Check sheet for the modelled part. Datum: model origin and axes. Units: mm. Round coordinates to 2 decimals unless told otherwise and drop trailing zeros. Write each loop counter-clockwise with the first axis right and the second up, starting at its lowest first coordinate (ties: lowest second). Pieces come first, ordered by that corner, then holes. Notation, with made-up numbers: (17.5, -14.5) -> (24.5, -14.5) arc R8 ccw to (24.5, -4.5) -> close; hole circle Ø2 at (44, 6.5). An arc over 180 degrees is marked (long way). One line per item, written item: value.
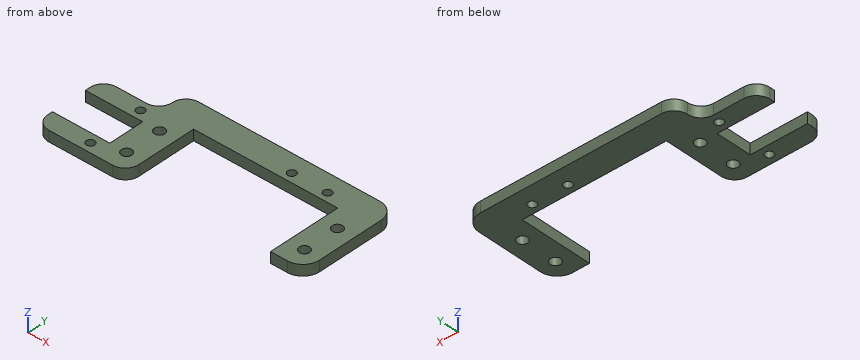
from build123d import *

# Parameters (mm, degrees)
BOSS_EXTRUDE7_DEPTH = 3
SKETCH12_R          = 1.15
CUT_EXTRUDE3_DEPTH  = 70.389048127
SKETCH11_R          = 1.45
CUT_EXTRUDE4_DEPTH  = 70.389048127
SKETCH13_R          = 1.15
CUT_EXTRUDE5_DEPTH  = 70.389048127
FILLET1_R           = 4.7
FILLET2_R           = 3.8


with BuildPart() as part:
    # Sketch10 → Boss-Extrude7 (new body)
    with BuildSketch(Plane.XY):
        Polygon((17.4, 10.2), (57.6, 10.2), (57.6, -10.2), (67, -10.2), (67, 17.8), (8, 17.8), (8, 10.2), (-8, 10.2), (-8, 5), (8, 5), (8, -5), (-8, -5), (-8, -10.2), (17.4, -10.2), align=None)
    extrude(amount=-BOSS_EXTRUDE7_DEPTH)

    # Sketch12 → Cut-Extrude3 (cut, through all)
    with BuildSketch(Plane(origin=(0, 0, 0), x_dir=(-1, 0, 0), z_dir=(0, 0, -1))):
        with Locations((-52.5, 12.7)):
            Circle(SKETCH12_R)
        with Locations((-42.5, 12.7)):
            Circle(SKETCH12_R)
    extrude(amount=CUT_EXTRUDE3_DEPTH, mode=Mode.SUBTRACT)

    # Sketch11 → Cut-Extrude4 (cut, through all)
    with BuildSketch(Plane(origin=(0, 0, 0), x_dir=(-1, 0, 0), z_dir=(0, 0, -1))):
        with Locations((-62.3, -5)):
            Circle(SKETCH11_R)
        with Locations((-12.7, -5)):
            Circle(SKETCH11_R)
        with Locations((-12.7, 5)):
            Circle(SKETCH11_R)
        with Locations((-62.3, 5)):
            Circle(SKETCH11_R)
    extrude(amount=CUT_EXTRUDE4_DEPTH, mode=Mode.SUBTRACT)

    # Sketch13 → Cut-Extrude5 (cut, through all)
    with BuildSketch(Plane.XY):
        with Locations((5, 7.6)):
            Circle(SKETCH13_R)
        with Locations((5, -7.6)):
            Circle(SKETCH13_R)
    extrude(amount=-CUT_EXTRUDE5_DEPTH, mode=Mode.SUBTRACT)

    # Fillet1
    fillet1_edges = [part.edges().sort_by_distance(p)[0] for p in [
        (67, 17.8, -1.5),
        (67, -10.2, -1.5),
    ]]
    fillet(fillet1_edges, radius=FILLET1_R)

    # Fillet2
    fillet2_edges = [part.edges().sort_by_distance(p)[0] for p in [
        (17.4, -10.2, -1.5),
        (-8, -10.2, -1.5),
        (8, 17.8, -1.5),
        (8, 10.2, -1.5),
        (-8, 10.2, -1.5),
    ]]
    fillet(fillet2_edges, radius=FILLET2_R - 0.0001)  # a hair under: the kernel refuses the full size


solid = part.part
Item 1: Sectioned sample at A-A (x = 52.5). Enter the section's corners in (y, z).
Result set:
outline: (10.2, -3) -> (11.55, -3) -> (11.55, 0) -> (10.2, 0) -> close; (13.85, -3) -> (17.8, -3) -> (17.8, 0) -> (13.85, 0) -> close
Item 2: Sectioned sample at C-C (z = -2.25). State how many separate pieces and enclosed holes the cut face has, then the cut area to 3 significant figures.
Result set:
separate pieces: 1
enclosed holes: 8
area: 937 mm^2
Item 3: Material ranges on line 1 along Y through (x, z) = (12.7, -0.75); line 2 along Y through (x, z) = (2.5, -1.7); line 3 along X through (y, z) = (12.7, -1.5), recorded low to high.
Result set:
line 1: -10.2 to -6.45, -3.55 to 3.55, 6.45 to 17.8
line 2: -10.2 to -5, 5 to 10.2
line 3: 7.77 to 41.35, 43.65 to 51.35, 53.65 to 67
Item 4: Sectioned sample at B-B (y = -2.25). Enter the section's corners in (x, z), then the cut area to 3 significant figures.
Result set:
outline: (8, -3) -> (17.4, -3) -> (17.4, 0) -> (8, 0) -> close; (57.6, -3) -> (67, -3) -> (67, 0) -> (57.6, 0) -> close
area: 56.4 mm^2
Item 5: Depth check by flat-ended pin: pin 1 (2.5 mm diameter, centred on x = 62.3, y = -5, fed in from +Z); pin 2 (1.5 mm diameter, centred on x = 33, z = -2, fed in from -Y); pin 3 (0.9 mm diameter, centred on y = 0, z = -2, fed in from -X); pin 4 (3.5 mm diameter, centred on x = 42.5, y = 12.7, fed in from +Z). Enter the tip coordinate at first touch or a pass-through.
Result set:
pin 1: through
pin 2: y = 10.2
pin 3: x = 8
pin 4: z = 0
Item 6: Sectioned sample at D-D (x = 5). Enter the section's corners in (y, z).
Result set:
outline: (-10.2, -3) -> (-8.75, -3) -> (-8.75, 0) -> (-10.2, 0) -> close; (-6.45, -3) -> (-5, -3) -> (-5, 0) -> (-6.45, 0) -> close; (5, -3) -> (6.45, -3) -> (6.45, 0) -> (5, 0) -> close; (8.75, -3) -> (10.29, -3) -> (10.29, 0) -> (8.75, 0) -> close
